from build123d import *

# Parameters (mm, degrees)
BOSS_EXTRUDE1_DEPTH = 5
SKETCH9_R           = 5
CUT_EXTRUDE4_DEPTH  = 10
SKETCH10_W          = 45.027348062
SKETCH10_H          = 31.505755331
CUT_EXTRUDE5_DEPTH  = 10
SKETCH11_W          = 70
SKETCH11_H          = 95
BOSS_EXTRUDE2_DEPTH = 5
SKETCH12_R          = 5
CUT_EXTRUDE6_DEPTH  = 5
SKETCH13_W          = 70
SKETCH13_H          = 30
BOSS_EXTRUDE3_DEPTH = 5
BOSS_EXTRUDE4_DEPTH = 5


with BuildPart() as part:
    # Sketch1 → Boss-Extrude1 (new body)
    with BuildSketch(Plane.XY):
        with BuildLine():
            Line((5, 0), (70, 0))
            Line((70, 0), (70, -30))
            Line((70, -30), (70, -95))
            Line((70, -95), (40, -95))
            Line((40, -95), (40, -30))
            Line((40, -30), (5, -30))
            ThreePointArc((5, -30), (1.464466094, -28.535533906), (0, -25))
            Line((0, -25), (0, -5))
            ThreePointArc((0, -5), (1.464466094, -1.464466094), (5, 0))
        make_face()
    boss_extrude1 = extrude(amount=BOSS_EXTRUDE1_DEPTH)

    # Mirror4: Boss-Extrude1 across plane
    add(boss_extrude1.mirror(Plane.ZY.offset(-55)))

    # Sketch9 → Cut-Extrude4 (cut)
    with BuildSketch(Plane(origin=(0, 0, 0), x_dir=(-1, 0, 0), z_dir=(0, 0, -1))):
        with Locations((-95, -15)):
            Circle(SKETCH9_R)
    extrude(amount=-CUT_EXTRUDE4_DEPTH, mode=Mode.SUBTRACT)

    # Sketch10 → Cut-Extrude5 (cut)
    with BuildSketch(Plane(origin=(0, 0, 0), x_dir=(-1, 0, 0), z_dir=(0, 0, -1))):
        with Locations((-17.486325969, -14.247122335)):
            Rectangle(SKETCH10_W, SKETCH10_H)
    extrude(amount=-CUT_EXTRUDE5_DEPTH, mode=Mode.SUBTRACT)

    # Sketch11 → Boss-Extrude2 (add)
    with BuildSketch(Plane(origin=(0, 0, 0), x_dir=(-1, 0, 0), z_dir=(0, 0, -1))):
        with Locations((-75, -47.5)):
            Rectangle(SKETCH11_W, SKETCH11_H)
    extrude(amount=-BOSS_EXTRUDE2_DEPTH)

    # Sketch12 → Cut-Extrude6 (cut)
    with BuildSketch(Plane(origin=(0, 0, 0), x_dir=(-1, 0, 0), z_dir=(0, 0, -1))):
        with Locations((-55, -15)):
            Circle(SKETCH12_R)
    extrude(amount=-CUT_EXTRUDE6_DEPTH, mode=Mode.SUBTRACT)

    # Sketch13 → Boss-Extrude3 (add)
    with BuildSketch(Plane.XZ.offset(95)):
        with Locations((75, -10)):
            Rectangle(SKETCH13_W, SKETCH13_H)
    extrude(amount=BOSS_EXTRUDE3_DEPTH)

    # Sketch14 → Boss-Extrude4 (add)
    with BuildSketch(Plane(origin=(100, 0, 0), x_dir=(0, 0, -1), z_dir=(1, 0, 0))):
        Polygon((0, -70), (25, -95), (0, -95), align=None)
    extrude(amount=BOSS_EXTRUDE4_DEPTH)


solid = part.part
Input: part model. Units: mm. Frame: model coordinates. A direction names the side the tool comes from. Give positions to 0.01 mm unless a question says otherwise; leave off trailing zeros. Order: outer loops, then holes, each group sorted by start corner. A loop starts at its lowest first (then second) coordinate and runs counter-clockwise, first axis right, second up. Notation, with made-up numbers: M 54.25,10.25 L 73.25,10.25 A21 cw 73.25,15.25 Z; hole C 45.5,72 d6. An arc over 180 degrees is marked long. Answer as a JSON object with one key per item and string values.
1. Reachability of faces 4 (the flat face through (107, -95, -12)), 5 (the flat face through (70, -95, -12)), 6 (the flat face through (75, -49, 5)) from +Z, -Z, +X, -X, +Y, -Y: full face, straight path, thin tool, end or side. Return the list, or none.
Result sheet:
{"face 4": "-Z, +X, +Y", "face 5": "-Z, -X, +Y", "face 6": "+Z, +X, -X, +Y, -Y"}
2. Cut plane D-D, the plane y = -84.5. Output: boundary loops of the cut face in (x, z).
Result sheet:
{"outline": "M 40,0 L 100,0 L 100,-14.5 L 105,-14.5 L 105,0 L 110,0 L 110,5 L 40,5 Z"}
3. Cut plane A-A, the plane x = 55. Output: boundary loops of the cut face in (y, z), and give its area (3 significant figures).
Result sheet:
{"outline": "M -100,-25 L -95,-25 L -95,0 L -20,0 L -20,5 L -100,5 Z; M -10,0 L 0,0 L 0,5 L -10,5 Z", "area": "575 mm²"}
4. Ray query, line 1 (Y direction, x = 55, z = 1.25); line 2 (Z direction, x = 99.5, y = -34); line 3 (Y direction, x = 76.5, z = -9.5). Return the intervals inside material, ascending. Write a range as [from, to].
Result sheet:
{"line 1": "[-100, -20], [-10, 0]", "line 2": "[0, 5]", "line 3": "[-100, -95]"}
5. Cut plane C-C, the plane z = -6. Output: boundary loops of the cut face in (x, y), and give its area (3 significant figures).
Result sheet:
{"outline": "M 40,-100 L 110,-100 L 110,-95 L 105,-95 L 105,-76 L 100,-76 L 100,-95 L 40,-95 Z", "area": "445 mm²"}
6. Cut plane B-B, the plane y = -15. Output: boundary loops of the cut face in (x, z).
Result sheet:
{"outline": "M 40,0 L 50,0 L 50,5 L 40,5 Z; M 60,0 L 110,0 L 110,5 L 60,5 Z"}
7. First-contact query: P1, Ø12, axis at y = -73.5, z = -17, coming from the +X side; P2, Ø7.5, axis at x = 84, z = -17.5, coming from the +Y side; P3, Ø1, axis at x = 76.5, y = -23.5, coming from the -Z side. Flat tips, straight axial feed; report the tip coordinate or a pass-through.
Result sheet:
{"P1": "through", "P2": "y = -95", "P3": "z = 0"}
8. Pull-direction query (X, two-part tool) for faces 1 (the flat face through (75, -47, 0)), 2 (the flat face through (105, -88, -7)), 3 (the cylindrical face through (59, -18, 2)); classes: +X half, -X half, draft (parallel to the pull), parting line (faces both ways), or undercut.
Result sheet:
{"face 1": "draft", "face 2": "+X half", "face 3": "undercut"}
